Model file for the job. Use its own axes, mm. A direction names the side the tool comes from. Give positions to 0.01 mm unless a question says otherwise; leave off trailing zeros. Loops run counter-clockwise (first coordinate to the right, second up) from the corner with the lowest first, then second, coordinate; pieces in that order, holes last. Notation, with made-up numbers: M -11.5,18 L 15.5,18 A23 cw 15.5,50 Z; hole C 36,71.25 d11. An arc over 180 degrees is marked long. Answer in a Markdown table with one row per item.
```python
from build123d import *

# Parameters (mm, degrees)
BOSS_EXTRUDE1_DEPTH = 133.35
SKETCH3_OUTSIDE_W   = 35.09
SKETCH3_OUTSIDE_H   = 36.072
SKETCH3_OUTSIDE_R   = 3.175
CUT_EXTRUDE1_DEPTH  = 57.15
SKETCH4_OUTSIDE_W   = 35.09
SKETCH4_OUTSIDE_H   = 36.072
SKETCH4_OUTSIDE_R   = 3.175
CUT_EXTRUDE2_DEPTH  = 15.875


with BuildPart() as part:
    # Sketch2 → Boss-Extrude1 (new body)
    with BuildSketch(Plane.XY):
        Polygon((0, 3.666174209), (-3.175, 1.833087105), (-3.175, -1.833087105), (0, -3.666174209), (3.175, -1.833087105), (3.175, 1.833087105), align=None)
    extrude(amount=BOSS_EXTRUDE1_DEPTH)

    # Sketch3 outside → Cut-Extrude1 (cut)
    with BuildSketch(Plane.XY.offset(133.35)):
        Rectangle(SKETCH3_OUTSIDE_W, SKETCH3_OUTSIDE_H)
        Circle(SKETCH3_OUTSIDE_R, mode=Mode.SUBTRACT)
    extrude(amount=-CUT_EXTRUDE1_DEPTH, mode=Mode.SUBTRACT)

    # Sketch4 outside → Cut-Extrude2 (cut)
    with BuildSketch(Plane(origin=(0, 0, 0), x_dir=(-1, 0, 0), z_dir=(0, 0, -1))):
        Rectangle(SKETCH4_OUTSIDE_W, SKETCH4_OUTSIDE_H)
        Circle(SKETCH4_OUTSIDE_R, mode=Mode.SUBTRACT)
    extrude(amount=-CUT_EXTRUDE2_DEPTH, mode=Mode.SUBTRACT)


solid = part.part
```
Q1. Probe probe 1 along X at (y, z) = (2.75, 78); probe 2 along Y at (x, z) = (-3, 46); probe 3 along X at (y, z) = (1.75, 120.5). List the from-to ranges inside material, lowest first.
Reported:
| item | result |
|---|---|
| probe 1 | -1.59 to 1.59 |
| probe 2 | -1.93 to 1.93 |
| probe 3 | -2.65 to 2.65 |
Q2. 3-axis set-ups, long thin cutter, end or side, ignore diameter. For faces 4 (the face through (-1.57, 2.76, 45.62)), 5 (the face through (0.69, -3.1, 7.83)), 6 (the face through (-0.69, -3.1, 105.18)): which of +Z, -Z, +X, -X, +Y, -Y reach the whole face in a straight line?
Reported:
| item | result |
|---|---|
| face 4 | +Z, -Z, -X, +Y |
| face 5 | -Z |
| face 6 | +Z |
Q3. Saw through at A-A (z = 22.5). Give the cut face in (x, y) (3 decimals).
Reported:
| item | result |
|---|---|
| outline | M -3.175,-1.833 L 0,-3.666 L 3.175,-1.833 L 3.175,1.833 L 0,3.666 L -3.175,1.833 Z |
Q4. Saw through at B-B (z = 86). Give the cut face in (x, y) (3 decimals), and give its area (3 significant figures).
Reported:
| item | result |
|---|---|
| outline | C 0,0 d6.35 |
| area | 31.7 mm² |
Q5. Drop a flat-ended pin along its axis: pin 1 (1 mm diameter, centred on x = 0, z = 94.5, fed in from +Y) (3 decimals). Give the stop position or say it passes through.
Reported:
| item | result |
|---|---|
| pin 1 | y = 3.175 |
Q6. Mould opens along Z. For faces 1 (the face through (0, 0, 0)), 2 (the face through (3.175, 0, 46)), 3 (the face through (0, 0, 133.35)) say: released by +Z, released by -Z, zero draft, split by the parting line, or undercut.
Reported:
| item | result |
|---|---|
| face 1 | released by -Z |
| face 2 | zero draft |
| face 3 | released by +Z |
